The listing builds one solid part. Answer for the finished solid, in the listing's coordinates (mm). A direction names the side the tool comes from. Give positions to 0.01 mm unless a question says otherwise; leave off trailing zeros. Order: outer loops, then holes, each group sorted by start corner. A loop starts at its lowest first (then second) coordinate and runs counter-clockwise, first axis right, second up. Notation, with made-up numbers: (75, 88) - (101, 88) arc R13 cw to (101, 110) - close; hole circle Ø2 at (36, -8.75). An arc over 180 degrees is marked (long way). Use a Markdown table: item, result. Add a question column.
1) Straight lines are drawn through the part: line 1 (Y direction, x = 0, z = 8.5); line 2 (Z direction, x = -2.5, y = -2.5); line 3 (Y direction, x = -1.75, z = 5.25). For each, find the intervals that lie inside material, in ascending order.
2) For faces 4 (the face through (3.09, -1.75, 0.2)), 5 (the face through (2, 3, 0.4)), determine the directions among +Z, -Z, +X, -X, +Y, -Y from which every point of the face is accessible in a straight line to the end or side of a thin tool.
3) Find section A-A, the plane x = 0. Determine the outline of the cut face in (y, z).
4) Find section C-C, the plane y = 3.25. Determine the outline of the cut face in (x, z), plus the area to 3 significant figures.
5) Find section B-B, the plane z = 4.5. Determine the outline of the cut face in (x, y).
6) The mould has two halves that part along Y. Classify faces 1 (the face through (-3.06, -1.8, 0.2)), 2 (the face through (-0.54, -2.44, 7.15)), 3 (the face through (3.06, 1.8, 0.2)): released by +Y, released by -Y, zero draft, split by the parting line, or undercut.
7) Flat-ended cylindrical pins translate along their axes: pin 1 (1.5 mm diameter, centred on x = 0, z = 11, fed in from -Y); pin 2 (3 mm diameter, centred on x = 1, z = 8.5, fed in from +Y); pin 3 (1.5 mm diameter, centred on y = -2, z = 2.5, fed in from -X); pin 4 (1 mm diameter, centred on x = -1.5, y = -0.5, fed in from +Z). Find the tip coordinate at first contact, or state that the pin passes through.
Autodesk Inventor part; units mm, degrees
ref_plane "YZ Plane" through (0, 0, 0) normal (1, 0, 0) x (0, 1, 0)
ref_plane "XZ Plane" through (0, 0, 0) normal (0, 1, 0) x (-1, 0, 0)
ref_plane "XY Plane" through (0, 0, 0) normal (0, 0, 1) x (1, 0, 0)
sketch "Sketch1" plane through (0, 0, 0) normal (0, 0, 1) x (1, 0, 0)
  line L0 (2.0496, 3.55) -> (4.0992, 0)
  line L1 (4.0992, 0) -> (2.0496, -3.55)
  line L2 (2.0496, -3.55) -> (-2.0496, -3.55)
  line L3 (-2.0496, -3.55) -> (-4.0992, 0)
  line L4 (-4.0992, 0) -> (-2.0496, 3.55)
  line L5 (-2.0496, 3.55) -> (2.0496, 3.55)
  point P0 (0, 0)
  dimension "d0" = 7.1
extrude "Extrusion1" add sketch "Sketch1" along normal blind 0.4
sketch "Sketch2" plane through (0, 0, 0.4) normal (0, 0, 1) x (1, 0, 0)
  circle A0 centre (0, 0) radius 3.4
  dimension "d3" = 6.8
extrude "Extrusion2" add sketch "Sketch2" along normal blind 14
sketch "Sketch3" plane through (0, 0, 14.4) normal (0, 0, 1) x (1, 0, 0)
  circle A0 centre (0, 0) radius 3.4
  circle A1 centre (0, 0) radius 2.5
  dimension "d6" = 5
extrude "Extrusion3" cut sketch "Sketch3" against normal blind 15 contours A1
chamfer "Chamfer1" distance 0.3 angle 45 1 edges at (-2.5, 0, 14.4)
thread "Thread1"
properties part number "Вытяжная заклепка_Р-Ш-М5-Ум" material "Сталь низкоуглеродистая"
The answers:
| question | item | result |
|---|---|---|
| 1 | line 1 | -3.4 to -2.5, 2.5 to 3.4 |
| 1 | line 2 | 0 to 0.4 |
| 1 | line 3 | -2.92 to -1.79, 1.79 to 2.92 |
| 2 | face 4 | +Z, -Z, +X, -Y |
| 2 | face 5 | +Z |
| 3 | outline | (-3.55, 0) - (-2.5, 0) - (-2.5, 14.1) - (-2.8, 14.4) - (-3.4, 14.4) - (-3.4, 0.4) - (-3.55, 0.4) - close; (2.5, 0) - (3.55, 0) - (3.55, 0.4) - (3.4, 0.4) - (3.4, 14.4) - (2.8, 14.4) - (2.5, 14.1) - close |
| 4 | outline | (-2.22, 0) - (2.22, 0) - (2.22, 0.4) - (1, 0.4) - (1, 14.4) - (-1, 14.4) - (-1, 0.4) - (-2.22, 0.4) - close |
| 4 | area | 29.7 mm2 |
| 5 | outline | circle Ø6.8 at (0, 0); hole circle Ø5 at (0, 0) |
| 6 | face 1 | released by -Y |
| 6 | face 2 | undercut |
| 6 | face 3 | released by +Y |
| 7 | pin 1 | y = -3.4 |
| 7 | pin 2 | y = 3.4 |
| 7 | pin 3 | x = -3.16 |
| 7 | pin 4 | through |
